Here's how the part is built. I have some questions about the finished solid (model axes, mm). Face numbers are marked on the shaded views. A direction names the side the tool comes from. Coordinates: 2 decimals unless noted, no trailing zeros. Loops run counter-clockwise (first coordinate to the right, second up) from the corner with the lowest first, then second, coordinate; pieces in that order, holes last. Notation, with made-up numbers: (43, 56) -> (86, 56) arc R31 ccw to (86, 93) -> close; hole circle Ø3 at (75.5, 62.25). An arc over 180 degrees is marked (long way). Use CSV: the item, a comma, the result in double quotes. Start each with the question number.
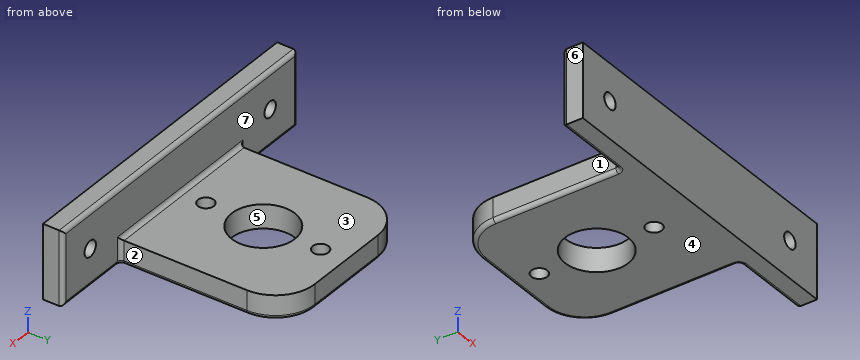
from build123d import *

# Parameters (mm, degrees)
SKETCH1_R           = 2
SKETCH1_R_2         = 8
BOSS_EXTRUDE1_DEPTH = 6
SKETCH2_W           = 12.7
SKETCH2_H           = 5.08
BOSS_EXTRUDE2_DEPTH = 82
FILLET1_R           = 10
FILLET2_R           = 10
FILLET4_R           = 1
SKETCH3_R           = 2
CUT_EXTRUDE1_DEPTH  = 6


with BuildPart() as part:
    # Sketch1 → Boss-Extrude1 (new body)
    with BuildSketch(Plane.XY):
        Polygon((0, 0), (82, 0), (82, 5.08), (62, 5.08), (62, 47.08), (20, 47.08), (20, 5.08), (0, 5.08), align=None)
        with Locations((41, 40.58)):
            Circle(SKETCH1_R, mode=Mode.SUBTRACT)
        with Locations((41, 11.58)):
            Circle(SKETCH1_R, mode=Mode.SUBTRACT)
        with Locations((41, 26.08)):
            Circle(SKETCH1_R_2, mode=Mode.SUBTRACT)
    extrude(amount=BOSS_EXTRUDE1_DEPTH)

    # Sketch2 → Boss-Extrude2 (add, through all)
    with BuildSketch(Plane(origin=(0, 0, 0), x_dir=(0, 0, -1), z_dir=(1, 0, 0))):
        with Locations((-12.35, 2.54)):
            Rectangle(SKETCH2_W, SKETCH2_H)
    extrude(amount=BOSS_EXTRUDE2_DEPTH)

    # Fillet1
    fillet1_edges = [part.edges().sort_by_distance(p)[0] for p in [
        (20, 47.08, 3),
    ]]
    fillet(fillet1_edges, radius=FILLET1_R)

    # Fillet2
    fillet2_edges = [part.edges().sort_by_distance(p)[0] for p in [
        (62, 47.08, 3),
    ]]
    fillet(fillet2_edges, radius=FILLET2_R)

    # Fillet4
    fillet4_edges = [part.edges().sort_by_distance(p)[0] for p in [
        (0, 5.08, 9.35),
        (20, 5.08, 3),
        (62, 5.08, 3),
        (82, 5.08, 9.35),
        (41, 5.08, 6),
        (41, 5.08, 18.7),
        (20, 21.08, 0),
        (22.928932188, 44.151067812, 0),
        (41, 47.08, 0),
        (59.071067812, 44.151067812, 0),
        (10, 5.08, 0),
        (62, 21.08, 0),
        (72, 5.08, 0),
    ]]
    fillet(fillet4_edges, radius=FILLET4_R)

    # Sketch3 → Cut-Extrude1 (cut)
    with BuildSketch(Plane(origin=(0, 0, 0), x_dir=(1, 0, 0), z_dir=(0, 1, 0))):
        with Locations((9.5, -9.35)):
            Circle(SKETCH3_R)
        with Locations((72.5, -9.35)):
            Circle(SKETCH3_R)
    extrude(amount=CUT_EXTRUDE1_DEPTH, mode=Mode.SUBTRACT)


solid = part.part
1) Thinking about a two-plate mould opening in Y: for the marked faces 5, 6 and 7, which applies, pulls with the +Y half, pulls with the -Y half, needs draft (parallel to the pull), parting line crosses it, or undercut?
2) I want a section at A-A, the plane z = 9.35. Please give me the cut outline in (x, y), plus the area to 3 significant figures.
3) For P1, Ø4, axis at y = 29, z = 2.5, coming from the +X side; P2, Ø8, axis at x = 16, z = 16.5, coming from the +Y side; P3, Ø2, axis at y = 22, z = 2, coming from the -X side, each with a flat end and sliding along its axis, tell me the tip position at first contact or that it passes through.
4) I want a section at D-D, the plane z = 3.5. Please give me the cut outline in (x, y).
5) Please list where these lines run through material, in increasing order: L1, parallel to Y at x = 41, z = 4.6; L2, parallel to Z at x = 9.5, y = 1.95; L3, parallel to Y at x = 42.5, z = 3.5. Write a range as [from, to].
6) I want a section at B-B, the plane y = 11.58. Please give me the cut outline in (x, z), plus the area to 3 significant figures.
7) Which directions (+Z, -Z, +X, -X, +Y, -Y) give clear straight access to the entire face, cutting with the end or side of a thin tool? Please do the marked faces 1, 2, 3 and 4.
8) I want a section at C-C, the plane x = 41. Please give me the cut outline in (y, z).
Return value:
1,face 5,"undercut"
1,face 6,"needs draft"
1,face 7,"pulls with the +Y half"
2,outline,"(0, 0) -> (7.5, 0) -> (7.5, 5.08) -> (1, 5.08) arc R1 ccw to (0, 4.08) -> close; (11.5, 0) -> (70.5, 0) -> (70.5, 5.08) -> (11.5, 5.08) -> close; (74.5, 0) -> (82, 0) -> (82, 4.08) arc R1 ccw to (81, 5.08) -> (74.5, 5.08) -> close"
2,area,"375 mm²"
3,P1,"stops at x = 62"
3,P2,"stops at y = 5.08"
3,P3,"stops at x = 20"
4,outline,"(0, 0) -> (82, 0) -> (82, 4.08) arc R1 ccw to (81, 5.08) -> (63, 5.08) arc R1 cw to (62, 6.08) -> (62, 37.08) arc R10 ccw to (52, 47.08) -> (30, 47.08) arc R10 ccw to (20, 37.08) -> (20, 6.08) arc R1 cw to (19, 5.08) -> (1, 5.08) arc R1 ccw to (0, 4.08) -> close; hole circle Ø16 at (41, 26.08); hole circle Ø4 at (41, 11.58); hole circle Ø4 at (41, 40.58)"
5,L1,"y = [0, 9.58], [13.58, 18.08], [34.08, 38.58], [42.58, 47.08]"
5,L2,"z = [0, 7.35], [11.35, 18.7]"
5,L3,"y = [0, 10.26], [12.9, 18.22], [33.94, 39.26], [41.9, 47.08]"
6,outline,"(20, 1) arc R1 ccw to (21, 0) -> (39, 0) -> (39, 6) -> (20, 6) -> close; (43, 0) -> (61, 0) arc R1 ccw to (62, 1) -> (62, 6) -> (43, 6) -> close"
6,area,"228 mm²"
7,face 1,"+Z, -Z, -X, +Y"
7,face 2,"+Z, -Z, +X, +Y"
7,face 3,"+Z, +X, -X, +Y"
7,face 4,"-Z, +X, -X, +Y, -Y"
8,outline,"(0, 0) -> (9.58, 0) -> (9.58, 6) -> (6.08, 6) arc R1 cw to (5.08, 7) -> (5.08, 17.7) arc R1 ccw to (4.08, 18.7) -> (0, 18.7) -> close; (13.58, 0) -> (18.08, 0) -> (18.08, 6) -> (13.58, 6) -> close; (34.08, 0) -> (38.58, 0) -> (38.58, 6) -> (34.08, 6) -> close; (42.58, 0) -> (46.08, 0) arc R1 ccw to (47.08, 1) -> (47.08, 6) -> (42.58, 6) -> close"
